Autodesk Fusion 360 part; units mm, degrees
sketch "Sketch1" plane through (0, 0, 0) normal (0, 0, 1) x (1, 0, 0)
  line L0 (0, 0) -> (50, 0)
  line L1 (50, 0) -> (50, 30)
  line L2 (50, 30) -> (0, 30)
  line L3 (0, 30) -> (0, 0)
  dimension "d1" = 50
  dimension "d2" = 30
extrude "Extrude1" add sketch "Sketch1" along normal blind 2
fillet "Fillet1" radius 1 1 faces at (16.6667, 20, 2)
sketch "Sketch2" plane through (0, 0, 2) normal (0, 0, 1) x (-1, 0, 0)
  line L0 (-49, -1) -> (-49, -29)
  line L1 (-49, -29) -> (-1, -29)
  line L2 (-1, -29) -> (-1, -1)
  line L3 (-1, -1) -> (-49, -1)
  circle A0 centre (-5, -15) radius 1
  circle A1 centre (-45, -15) radius 1
  line L4 (0, -30) -> (0, 0)
  line L5 (-50, -30) -> (0, -30)
  dimension "d7" = 2
  dimension "d8" = 2
  dimension "d9" = 40
  dimension "d10" = 5
  dimension "d11" = 15
extrude "Extrude2" cut sketch "Sketch2" against normal blind 1 contours A0 | A1
sketch "Sketch3" plane through (0, 0, 2) normal (0, 0, 1) x (-1, 0, 0)
  circle A0 centre (-45, -15) radius 1
  circle A1 centre (-5, -15) radius 1
  line L0 (-49, -1) -> (-49, -29)
  line L1 (-49, -29) -> (-1, -29)
  line L2 (-1, -29) -> (-1, -1)
  line L3 (-1, -1) -> (-49, -1)
  circle A2 centre (-5, -15) radius 2
  circle A3 centre (-45, -15) radius 2
  dimension "d14" = 4
  dimension "d15" = 4
extrude "Extrude4" cut sketch "Sketch3" against normal blind 11 contours A0 | A1
extrude "Extrude5" cut sketch "Sketch3" against normal blind 1 contours A2 | A3
extrude "Extrude3" [suppressed]
Check sheet for the modelled part. Datum: model origin and axes. Units: mm. A direction names the side the tool comes from. Coordinates: 2 decimals unless noted, no trailing zeros. Loops run counter-clockwise (first coordinate to the right, second up) from the corner with the lowest first, then second, coordinate; pieces in that order, holes last.
1) Gauge pin test, flat end, axial feed: pin 1 (2.5 mm diameter, centred on x = 5, y = 15, fed in from +Z). Record the tip position at first contact, or that the pin passes through.
2) Release check for a two-part mould opening along X. For faces 1 (the face through (25.3, 30, 0.5)), 2 (the face through (49.699, 15.21, 1.715)), 3 (the face through (0.301, 14.79, 1.715)), 4 (the face through (5.217, 15.976, 0.507)) record: released by +X, released by -X, zero draft, split by the parting line, or undercut.
3) Access from +Z, -Z, +X, -X, +Y, -Y to the whole of each face (thin tool, end or side, straight path). Record for faces 5 (the face through (45.26, 13.017, 1.507)), 6 (the face through (50, 14.8, 0.5)).
4) Material ranges on probe 1 along X at (y, z) = (15, 0.5); probe 2 along X at (y, z) = (15, 1.7); probe 3 along Y at (x, z) = (45, 0.6), recorded low to high.
5) Sectioned sample at B-B (x = 5). Record the boundary of the cut face in (y, z).
6) Sectioned sample at C-C (z = 1.6). Record the boundary of the cut face in (x, y), and give its area (3 significant figures).
7) Sectioned sample at A-A (y = 15). Record the boundary of the cut face in (x, z).
Check sheet entries:
1. pin 1: stops at z = 1
2. face 1: zero draft
2. face 2: released by +X
2. face 3: released by -X
2. face 4: undercut
3. face 5: +Z
3. face 6: +Z, -Z, +X, +Y, -Y
4. probe 1: x = 0 to 4, 6 to 44, 46 to 50
4. probe 2: x = 0.29 to 3, 7 to 43, 47 to 49.71
4. probe 3: y = 0 to 14, 16 to 30
5. outline: (0, 0) - (14, 0) - (14, 1) - (13, 1) - (13, 2) - (1, 2) arc R1 ccw to (0, 1) - close; (16, 0) - (30, 0) - (30, 1) arc R1 ccw to (29, 2) - (17, 2) - (17, 1) - (16, 1) - close
6. outline: (0.2, 0.2) - (49.8, 0.2) - (49.8, 29.8) - (0.2, 29.8) - close; hole circle Ø4 at (5, 15); hole circle Ø4 at (45, 15)
6. area: 1,440 mm2
7. outline: (0, 0) - (4, 0) - (4, 1) - (3, 1) - (3, 2) - (1, 2) arc R1 ccw to (0, 1) - close; (6, 0) - (44, 0) - (44, 1) - (43, 1) - (43, 2) - (7, 2) - (7, 1) - (6, 1) - close; (46, 0) - (50, 0) - (50, 1) arc R1 ccw to (49, 2) - (47, 2) - (47, 1) - (46, 1) - close
